Job drawing, mm, ordinate dimensions from the low corner. One solid piece. Coordinates: 2 decimals unless noted, no trailing zeros. Write each loop counter-clockwise with the first axis right and the second up, starting at its lowest first coordinate (ties: lowest second). Pieces come first, ordered by that corner, then holes.
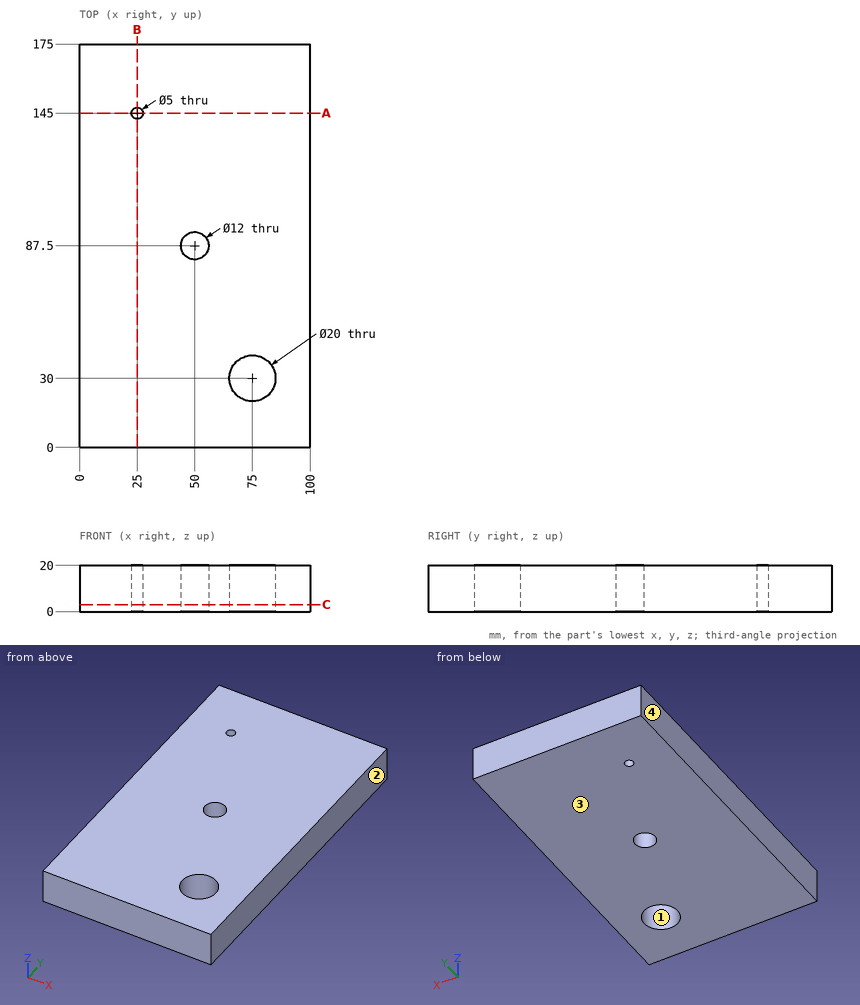
1. Saw through at B-B on x = 25. List the corners of the cut face in (y, z), plus the area to 3 significant figures.
Computed values:
outline: (0, 0) - (142.5, 0) - (142.5, 20) - (0, 20) - close; (147.5, 0) - (175, 0) - (175, 20) - (147.5, 20) - close
area: 3,400 mm2
2. Probe line 1 along Y through (x, z) = (75, 14.5); line 2 along Y through (x, z) = (50, 14.75); line 3 along X through (y, z) = (145, 14.5). List the from-to ranges inside material, lowest first.
Computed values:
line 1: y = 0 to 20, 40 to 175
line 2: y = 0 to 81.5, 93.5 to 175
line 3: x = 0 to 22.5, 27.5 to 100
3. Mould opens along X. For the marked faces 1, 2, 3 and 4 say: +X half, -X half, draft (parallel to the pull), parting line (faces both ways), or undercut.
Computed values:
face 1: undercut
face 2: +X half
face 3: draft
face 4: -X half
4. Saw through at C-C on z = 3. List the corners of the cut face in (x, y), plus the area to 3 significant figures.
Computed values:
outline: (0, 0) - (100, 0) - (100, 175) - (0, 175) - close; hole circle Ø5 at (25, 145); hole circle Ø12 at (50, 87.5); hole circle Ø20 at (75, 30)
area: 17,100 mm2
5. Saw through at A-A on y = 145. List the corners of the cut face in (x, z).
Computed values:
outline: (0, 0) - (22.5, 0) - (22.5, 20) - (0, 20) - close; (27.5, 0) - (100, 0) - (100, 20) - (27.5, 20) - close
